from build123d import *

# Parameters (mm, degrees)
SKETCH1_W                = 31.2
SKETCH1_H                = 15
SKETCH1_R                = 1.375
BOSS_EXTRUDE1_DEPTH      = 2
SKETCH2_W                = 3
SKETCH2_H                = 5
BOSS_EXTRUDE2_DEPTH      = 26.54
BOSS_EXTRUDE3_DEPTH      = 5
BOSS_EXTRUDE3_DEPTH_BACK = 10
SKETCH3_W                = 3
SKETCH3_H                = 12
BOSS_EXTRUDE4_DEPTH      = 3
BOSS_EXTRUDE5_DEPTH      = 3


with BuildPart() as part:
    # Sketch1 → Boss-Extrude1 (new body)
    with BuildSketch(Plane(origin=(0, 0, 0), x_dir=(1, 0, 0), z_dir=(0, 1, 0))):
        with Locations((15.6, 7.5)):
            Rectangle(SKETCH1_W, SKETCH1_H)
        with Locations(Location((15.6, 10, 0), (0, 0, 270))):
            Circle(SKETCH1_R, mode=Mode.SUBTRACT)
        with Locations(Location((10.6, 5, 0), (0, 0, 270))):
            Circle(SKETCH1_R, mode=Mode.SUBTRACT)
        with Locations(Location((20.6, 5, 0), (0, 0, 270))):
            Circle(SKETCH1_R, mode=Mode.SUBTRACT)
    extrude(amount=BOSS_EXTRUDE1_DEPTH)

    # Sketch2 → Boss-Extrude2 (add)
    with BuildSketch(Plane(origin=(0, 2, 0), x_dir=(1, 0, 0), z_dir=(0, 1, 0))):
        with Locations((1.5, 12.5)):
            Rectangle(SKETCH2_W, SKETCH2_H)
        with Locations((29.7, 12.5)):
            Rectangle(SKETCH2_W, SKETCH2_H)
    extrude(amount=BOSS_EXTRUDE2_DEPTH)

    # Sketch3 → Boss-Extrude3 (add, two sides: drawn at the far end of the back side and taken through both)
    with BuildSketch(Plane(origin=(0, 0, -15), x_dir=(-1, 0, 0), z_dir=(0, 0, -1)).offset(-BOSS_EXTRUDE3_DEPTH_BACK)):
        with Locations((-29.7, 19.54)):
            Rectangle(SKETCH3_W, SKETCH3_H)
        with Locations((-1.5, 19.54)):
            Rectangle(SKETCH3_W, SKETCH3_H)
    extrude(amount=BOSS_EXTRUDE3_DEPTH + BOSS_EXTRUDE3_DEPTH_BACK)

    # Sketch5 → Boss-Extrude4 (add)
    with BuildSketch(Plane(origin=(31.2, 0, 0), x_dir=(0, 0, -1), z_dir=(1, 0, 0))):
        Polygon((10, 4), (6.535898385, 2), (10, 2), align=None)
    extrude(amount=-BOSS_EXTRUDE4_DEPTH)

    # Sketch6 → Boss-Extrude5 (add)
    with BuildSketch(Plane(origin=(0, 0, 0), x_dir=(0, 0, -1), z_dir=(1, 0, 0))):
        Polygon((10, 4), (6.535898385, 2), (10, 2), align=None)
    extrude(amount=BOSS_EXTRUDE5_DEPTH)


solid = part.part
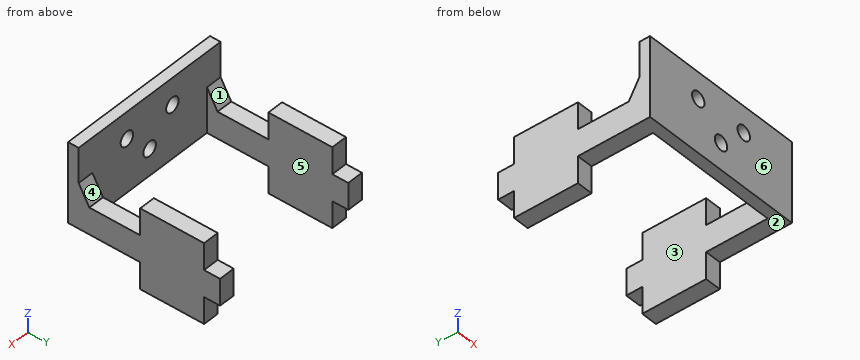
Can you work these out from the model? Positions are in its coordinate system, mm. Face numbers are marked on the shaded views. A direction names the side the tool comes from. Give positions to 0.01 mm unless a question says otherwise; leave off trailing zeros. Loops run counter-clockwise (first coordinate to the right, second up) from the corner with the lowest first, then second, coordinate; pieces in that order, holes last. Notation, with made-up numbers: (68.25, 5) -> (86.25, 5) arc R31 ccw to (86.25, 30) -> close; hole circle Ø1 at (85, -39). An arc over 180 degrees is marked (long way). Return JSON: item names as keys, results as strings.
Q1. For pin 1 Ø6 at (x, z) = (9, -4) entering from +Y; pin 2 Ø0.9 at (x, z) = (29.5, -16.5) entering from +Y; pin 3 Ø3.5 at (x, y) = (29.5, 10) entering from +Z, each with a flat end and sliding along its axis, tell me the tip position at first contact or that it passes through.
Checks:
{"pin 1": "stops at y = 2", "pin 2": "stops at y = 25.54", "pin 3": "stops at z = -10"}
Q2. I want a section at B-B, the plane x = 20.6. List the corners of the cut face in (y, z) for me (3 decimals).
Checks:
{"outline": "(0, -15) -> (2, -15) -> (2, -6.375) -> (0, -6.375) -> close; (0, -3.625) -> (2, -3.625) -> (2, 0) -> (0, 0) -> close"}
Q3. I want a section at C-C, the plane z = -12. List the corners of the cut face in (x, y) for me, then the cut area to 3 significant figures.
Checks:
{"outline": "(0, 0) -> (31.2, 0) -> (31.2, 28.54) -> (28.2, 28.54) -> (28.2, 2) -> (3, 2) -> (3, 28.54) -> (0, 28.54) -> close", "area": "222 mm2"}
Q4. I want a section at D-D, the plane x = 24. List the corners of the cut face in (y, z) for me.
Checks:
{"outline": "(0, -15) -> (2, -15) -> (2, 0) -> (0, 0) -> close"}
Q5. I want a section at A-A, the plane y = 20.5. List the corners of the cut face in (x, z) for me.
Checks:
{"outline": "(0, -20) -> (3, -20) -> (3, -5) -> (0, -5) -> close; (28.2, -20) -> (31.2, -20) -> (31.2, -5) -> (28.2, -5) -> close"}
Q6. I need wall thicknesses on probe 1 along X at (y, z) = (0.9, -5) (3 decimals); probe 2 along X at (y, z) = (18.75, -12); probe 3 along X at (y, z) = (0.5, -10) (3 decimals). Which ranges of each line are inside material? Lowest first, please.
Checks:
{"probe 1": "x = 0 to 9.225, 11.975 to 19.225, 21.975 to 31.2", "probe 2": "x = 0 to 3, 28.2 to 31.2", "probe 3": "x = 0 to 14.225, 16.975 to 31.2"}
Q7. We'd pull the mould along Y, two halves only. Please class the marked faces 4, 5 and 6: released by +Y, released by -Y, zero draft, split by the parting line, or undercut.
Checks:
{"face 4": "undercut", "face 5": "zero draft", "face 6": "released by -Y"}
Q8. On a 3-axis mill with a long thin cutter (end or side, diameter ignored), from which of +Z, -Z, +X, -X, +Y, -Y can I reach the whole of each face in a straight line? I mean the marked faces 1, 2 and 3. Say none if no direction works.
Checks:
{"face 1": "+Z, +X, -X", "face 2": "-Z, +X, -X, -Y", "face 3": "+Z, -Z, +Y"}
